The listing builds one solid part. Answer for the finished solid, in the listing's coordinates (mm). A direction names the side the tool comes from. Coordinates: 2 decimals unless noted, no trailing zeros. Loops run counter-clockwise (first coordinate to the right, second up) from the corner with the lowest first, then second, coordinate; pieces in that order, holes last. Notation, with made-up numbers: (35.5, 37.25) - (73.5, 37.25) arc R23 cw to (73.5, 62.25) - close; hole circle Ø7 at (86, -16). An arc over 180 degrees is marked (long way). Put each result on its own line as item: value.
```python
from build123d import *

# Parameters (mm, degrees)
F0_R     = 32.5
F1_DEPTH = 2
F2_R     = 31.3
F2_R_2   = 8
F3_DEPTH = 1
F5_DEPTH = 1
F6_COUNT = 25


with BuildPart() as f1:
    # F0 (on Top) → F1 (new body)
    with BuildSketch(Plane.XY):
        Circle(F0_R)
    extrude(amount=F1_DEPTH)

    # F2 (on face) → F3 (cut)
    with BuildSketch(Plane.XY.offset(2)):
        Circle(F2_R)
        Circle(F2_R_2, mode=Mode.SUBTRACT)
    extrude(amount=-F3_DEPTH, mode=Mode.SUBTRACT)

    # F4 (on face) → F5 (join, through all)
    with BuildSketch(Plane.XY.offset(1)):
        with BuildLine():
            ThreePointArc((-0.6, 9.981984), (0, 10), (0.6, 9.981984))
            Line((0.6, 9.981984), (0.2, 30))
            Line((0.2, 30), (0, 30))
            Line((0, 30), (-0.2, 30))
            Line((-0.2, 30), (-0.6, 9.981984))
        make_face()
    extrude(amount=F5_DEPTH)

    # F6: F1 ×25 about axis
    f6_axis = Axis((0, 0, 0), (0, 0, -1))


with BuildPart() as f1_1:
    add(f1.part)
    for i in range(1, F6_COUNT):
        add(f1.part.rotate(f6_axis, i * 360 / F6_COUNT))


solid = f1_1.part
```
1) The part is cut by section B-B (y = -26). Give the vertices of the cut face in (x, z), and give its area (3 significant figures).
Found:
outline: (-19.5, 0) - (19.5, 0) - (19.5, 2) - (17.43, 2) - (17.43, 1) - (10.55, 1) - (10.55, 2) - (10.03, 2) - (10.03, 1) - (3.56, 1) - (3.56, 2) - (3.01, 2) - (3.01, 1) - (-3.01, 1) - (-3.01, 2) - (-3.56, 2) - (-3.56, 1) - (-10.03, 1) - (-10.03, 2) - (-10.55, 2) - (-10.55, 1) - (-17.43, 1) - (-17.43, 2) - (-19.5, 2) - close
area: 45.3 mm^2
2) This flat-tipped pin is pushed along its axis until it touches: pin 1 (1 mm diameter, centred on y = -17.5, z = 0.5, fed in from -X). Where does it stop, or does it pass through?
Found:
pin 1: stops at x = -27.7
3) The part is cut by section A-A (z = 1.35). State how many separate pieces and enclosed holes the cut face has, and give its area (3 significant figures).
Found:
separate pieces: 27
enclosed holes: 1
area: 842 mm^2
4) For a pull along Y with two mould halves and no side action, classify faces 3 (the face through (31, 9.76, 0.99)), 4 (the face through (-19.7, -4.162, 1.493)), 5 (the face through (-13.8, -11.4, 2)) as pulls with the +Y half, pulls with the -Y half, needs draft (parallel to the pull), parting line crosses it, or undercut.
Found:
face 3: parting line crosses it
face 4: undercut
face 5: needs draft
5) Straight lines are drawn through the part: L1, parallel to Y at x = 0, z = 1.4; L2, parallel to Y at x = -26, z = 1.6; L3, parallel to Z at x = 26.5, y = 5. For each, find the intervals that lie inside material, in ascending order. Write a range as [from, to].
Found:
L1: y = [-32.5, -31.3], [-8, 8], [10, 30], [31.3, 32.5]
L2: y = [-19.5, -17.43], [-12.48, -11.98], [-5.23, -4.68], [1.36, 1.91], [8.18, 8.71], [17.43, 19.5]
L3: z = [0, 1]
6) For faces 1 (the face through (2, -18, 2)), 2 (the face through (-7.682, -18.309, 1.493)), determine the directions among +Z, -Z, +X, -X, +Y, -Y from which every point of the face is accessible in a straight line to the end or side of a thin tool.
Found:
face 1: +Z, +X, -X, +Y, -Y
face 2: +Z
